Read the model definition and answer for the solid it produces. Units are mm, in the model's axes. A direction names the side the tool comes from. Give positions to 0.01 mm unless a question says otherwise; leave off trailing zeros. Loops run counter-clockwise (first coordinate to the right, second up) from the corner with the lowest first, then second, coordinate; pieces in that order, holes last. Notation, with made-up numbers: (23, 74.5) - (71, 74.5) arc R25 ccw to (71, 91.5) - close; hole circle Ø5 at (-33.75, 19). An arc over 180 degrees is marked (long way). Write item = value, one per line.
```python
from build123d import *

# Parameters (mm, degrees)
SKETCH2_W           = 305
SKETCH2_H           = 150
BOSS_EXTRUDE1_DEPTH = 6.375
SKETCH3_W           = 124
SKETCH3_H           = 3.5
CUT_EXTRUDE1_DEPTH  = 306
SKETCH4_W           = 197.5
SKETCH4_H           = 30
BOSS_EXTRUDE2_DEPTH = 55
BOSS_EXTRUDE3_DEPTH = 59.2
SKETCH6_W           = 73
SKETCH6_H           = 118
BOSS_EXTRUDE4_DEPTH = 27.3
BOSS_EXTRUDE5_DEPTH = 38.7
BOSS_EXTRUDE6_DEPTH = 60.9
SKETCH9_W           = 16
SKETCH9_H           = 150
BOSS_EXTRUDE7_DEPTH = 9
SKETCH10_W          = 170
SKETCH10_H          = 85
CUT_EXTRUDE2_DEPTH  = 40.7


with BuildPart() as part:
    # Sketch2 → Boss-Extrude1 (new body, symmetric)
    with BuildSketch(Plane(origin=(0, 0, 0), x_dir=(1, 0, 0), z_dir=(0, 1, 0))):
        Rectangle(SKETCH2_W, SKETCH2_H)
    extrude(amount=BOSS_EXTRUDE1_DEPTH, both=True)

    # Sketch3 → Cut-Extrude1 (cut, through all)
    with BuildSketch(Plane(origin=(152.5, 0, 0), x_dir=(0, 0, -1), z_dir=(1, 0, 0))):
        with Locations((0, 4.625)):
            Rectangle(SKETCH3_W, SKETCH3_H)
    extrude(amount=-CUT_EXTRUDE1_DEPTH, mode=Mode.SUBTRACT)

    # Sketch4 → Boss-Extrude2 (add)
    with BuildSketch(Plane.XY.offset(75)):
        with Locations((-23.75, 8.625)):
            Rectangle(SKETCH4_W, SKETCH4_H)
    extrude(amount=BOSS_EXTRUDE2_DEPTH)

    # Sketch5 → Boss-Extrude3 (add)
    with BuildSketch(Plane.ZY.offset(122.5)):
        with BuildLine():
            Line((84.426315846, -10.75), (114.823684154, -10.75))
            ThreePointArc((114.823684154, -10.75), (99.625, 33.25), (84.426315846, -10.75))
        make_face()
    extrude(amount=BOSS_EXTRUDE3_DEPTH)

    # Sketch6 → Boss-Extrude4 (add)
    with BuildSketch(Plane.XZ.offset(6.375)):
        with Locations((144.1, 16)):
            Rectangle(SKETCH6_W, SKETCH6_H)
    extrude(amount=BOSS_EXTRUDE4_DEPTH)

    # Sketch7 → Boss-Extrude5 (add)
    with BuildSketch(Plane.XY.offset(75)):
        Polygon((107.6, -33.675), (107.6, 2.325), (141.6, 2.325), (151.6, -10.675), (159.2, -10.675), (159.2, -33.675), align=None)
    extrude(amount=BOSS_EXTRUDE5_DEPTH)

    # Sketch8 → Boss-Extrude6 (add)
    with BuildSketch(Plane.XY.offset(113.7)):
        with BuildLine():
            Line((110.972997108, -36.825), (140.637791056, -36.825))
            ThreePointArc((140.637791056, -36.825), (125.805394082, 7.175), (110.972997108, -36.825))
        make_face()
    extrude(amount=BOSS_EXTRUDE6_DEPTH)

    # Sketch9 → Boss-Extrude7 (add)
    with BuildSketch(Plane.XZ.offset(6.375)):
        with Locations((-130.5, 0)):
            Rectangle(SKETCH9_W, SKETCH9_H)
        with Locations((99.6, 0)):
            Rectangle(SKETCH9_W, SKETCH9_H)
    extrude(amount=BOSS_EXTRUDE7_DEPTH)

    # Sketch10 → Cut-Extrude2 (cut, through all)
    with BuildSketch(Plane(origin=(0, 2.875, 0), x_dir=(1, 0, 0), z_dir=(0, 1, 0))):
        Rectangle(SKETCH10_W, SKETCH10_H)
    extrude(amount=-CUT_EXTRUDE2_DEPTH, mode=Mode.SUBTRACT)


solid = part.part
```
1) Each of these flat-tipped pins is pushed along its axis until it touches: P1, Ø10, axis at x = -3.5, z = 74, coming from the -Y side (3 decimals); P2, Ø4.5, axis at x = 39.5, y = -3.5, coming from the +Z side; P3, Ø9, axis at x = -154, z = 104.5, coming from the -Y side. Where does it stop, or does it pass through?
Output:
P1 = -6.375
P2 = 130
P3 = -10.75
2) A tool of negligible diameter and unlimited length cuts with its end or side. For faces 5 (the face through (2, 2.875, 56)), 6 (the face through (75, 8, 102)), 7 (the face through (159.2, -22, 94)), 8 (the face through (166, -6.375, 17)), from which of +Z, -Z, +X, -X, +Y, -Y can it reach the whole face along a straight path? Write none if from no direction.
Output:
face_5 = +X, -X, +Y
face_6 = +Z, +Y, -Y
face_7 = +Z, +X, +Y, -Y
face_8 = +Z, -Z, +X, +Y
3) A cutting plane is placed at A-A on x = -27.5. Determine the outline of the cut face in (y, z) (3 decimals).
Output:
outline = (-6.375, -75) - (6.375, -75) - (6.375, -62) - (2.875, -62) - (2.875, -42.5) - (-6.375, -42.5) - close; (-6.375, 42.5) - (2.875, 42.5) - (2.875, 62) - (6.375, 62) - (6.375, 75) - (23.625, 75) - (23.625, 130) - (-6.375, 130) - close
4) A cutting plane is placed at B-B on z = -38. Determine the outline of the cut face in (x, y) (3 decimals).
Output:
outline = (-152.5, -6.375) - (-138.5, -6.375) - (-138.5, -15.375) - (-122.5, -15.375) - (-122.5, -6.375) - (-85, -6.375) - (-85, 2.875) - (-152.5, 2.875) - close; (85, -6.375) - (91.6, -6.375) - (91.6, -15.375) - (107.6, -15.375) - (107.6, -33.675) - (180.6, -33.675) - (180.6, -6.375) - (152.5, -6.375) - (152.5, 2.875) - (85, 2.875) - close
5) Find the intervals of material crossed by probe 1 along Z at (x, y) = (102, -14.5); probe 2 along Z at (x, y) = (-46.5, 4); probe 3 along X at (y, z) = (-1, 126), in increasing order.
Output:
probe_1 = -75 to 75, 113.7 to 174.6
probe_2 = -75 to -62, 62 to 130
probe_3 = -122.5 to 75, 107.54 to 144.07
6) A cutting plane is placed at D-D on x = -144. Determine the outline of the cut face in (y, z) (3 decimals), then the cut area to 3 significant figures.
Output:
outline = (-10.75, 84.426) arc R24.625 ccw (long way) to (-10.75, 114.824) - close; (-6.375, -75) - (6.375, -75) - (6.375, -62) - (2.875, -62) - (2.875, 62) - (6.375, 62) - (6.375, 75) - (-6.375, 75) - close
area = 3,270 mm²
7) A cutting plane is placed at C-C on z = 52.5. Determine the outline of the cut face in (x, y) (3 decimals).
Output:
outline = (-152.5, -6.375) - (-138.5, -6.375) - (-138.5, -15.375) - (-122.5, -15.375) - (-122.5, -6.375) - (91.6, -6.375) - (91.6, -15.375) - (107.6, -15.375) - (107.6, -33.675) - (180.6, -33.675) - (180.6, -6.375) - (152.5, -6.375) - (152.5, 2.875) - (-152.5, 2.875) - close
8) The mould has two halves that part along Z. Classify faces 1 (the face through (-138.5, -11, -1)), 2 (the face through (-1, -2, 42.5)), 3 (the face through (125, -15, 174.6)), 4 (the face through (-2, -2, -75)): pulls with the +Z half, pulls with the -Z half, needs draft (parallel to the pull), parting line crosses it, or undercut.
Output:
face_1 = needs draft
face_2 = undercut
face_3 = pulls with the +Z half
face_4 = pulls with the -Z half
